from build123d import *

# Parameters (mm, degrees)
BOSS_EXTRUDE1_DEPTH = 1
SKETCH2_R           = 7.5
CUT_EXTRUDE1_DEPTH  = 26.455844123
FILLET1_R           = 5


with BuildPart() as part:
    # Sketch1 → Boss-Extrude1 (new body)
    with BuildSketch(Plane.XY):
        with BuildLine():
            Line((-17.972200756, -1), (17.972200756, -1))
            ThreePointArc((17.972200756, -1), (0, -18), (-17.972200756, -1))
        make_face()
    extrude(amount=BOSS_EXTRUDE1_DEPTH)

    # Sketch2 → Cut-Extrude1 (cut, through all)
    with BuildSketch(Plane.XY.offset(1)):
        Circle(SKETCH2_R)
    extrude(amount=-CUT_EXTRUDE1_DEPTH, mode=Mode.SUBTRACT)

    # Fillet1
    fillet1_edges = [part.edges().sort_by_distance(p)[0] for p in [
        (7.433034374, -1, 0.5),
        (-7.433034374, -1, 0.5),
    ]]
    fillet(fillet1_edges, radius=FILLET1_R)


solid = part.part
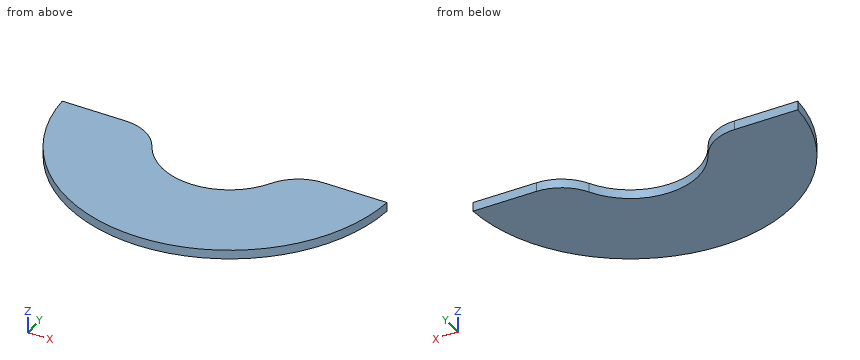
CAD build for the part. Positions are in the model's coordinates, mm. Round coordinates to 2 decimals unless told otherwise and drop trailing zeros. Loops run counter-clockwise (first coordinate to the right, second up) from the corner with the lowest first, then second, coordinate; pieces in that order, holes last. Notation, with made-up numbers: M 17,-2 L 50,-2 A19 cw 50,10 Z; hole C -38.75,8 d2. An arc over 180 degrees is marked long. One line per question, with ' | ' between items. Start each with the question number.
Item 1: Wall check: line 1 (X direction, y = -2, z = 0.6); line 2 (X direction, y = -12.75, z = 0.95); line 3 (Y direction, x = -11, z = 0.55). Give the ranges that are in metal, low to high.
Item 2: Cut at B-B, the plane z = 0.6. Write the cut outline in (x, y), plus the area to 3 significant figures.
Item 3: Cut at C-C, the plane x = 0. Write the cut outline in (y, z), plus the area to 3 significant figures.
Item 4: Cut at D-D, the plane y = -8.25. Write the cut outline in (x, z).
Item 5: Cut at A-A, the plane y = -4. Write the cut outline in (x, z), plus the area to 3 significant figures.
Item 6: Pin check, flat tip, straight feed: pin 1 Ø8 at (x, y) = (3, -4.5) entering from +Z. Stop position of the tip, or through.
Responses:
1) line 1: x = -17.89 to -7.97, 7.97 to 17.89 | line 2: x = -12.71 to 12.71 | line 3: y = -14.25 to -1
2) outline: M -17.97,-1 A18 ccw 17.97,-1 L 10.97,-1 A5 ccw 6.58,-3.6 A7.5 cw -6.58,-3.6 A5 ccw -10.97,-1 Z | area: 396 mm²
3) outline: M -18,0 L -7.5,0 L -7.5,1 L -18,1 Z | area: 10.5 mm²
4) outline: M -16,0 L 16,0 L 16,1 L -16,1 Z
5) outline: M -17.55,0 L -6.34,0 L -6.34,1 L -17.55,1 Z; M 6.34,0 L 17.55,0 L 17.55,1 L 6.34,1 Z | area: 22.4 mm²
6) pin 1: stops at z = 1
